For this review, take the finished solid that the model builds, in its own axes (mm). Face numbers are marked on the shaded views. A direction names the side the tool comes from. Coordinates: 2 decimals unless noted, no trailing zeros. Loops run counter-clockwise (first coordinate to the right, second up) from the corner with the lowest first, then second, coordinate; pieces in that order, holes last. Notation, with made-up numbers: M 36,-18.5 L 52,-18.5 A19 ccw 52,-12.5 Z; hole C 86.25,53.5 d8. An arc over 180 degrees is marked long. Put each result on its own line as item: value.
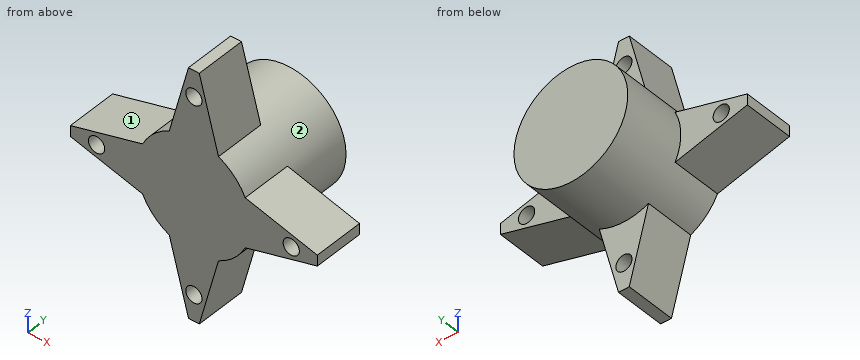
```python
from build123d import *

# Parameters (mm, degrees)
SKETCH1_R           = 7.895
BOSS_EXTRUDE1_DEPTH = 15.79
SKETCH2_R           = 1.125
BOSS_EXTRUDE2_DEPTH = 7


with BuildPart() as part:
    # Sketch1 → Boss-Extrude1 (new body)
    with BuildSketch(Plane(origin=(0, 0, 0), x_dir=(1, 0, 0), z_dir=(0, 1, 0))):
        Circle(SKETCH1_R)
    extrude(amount=BOSS_EXTRUDE1_DEPTH)

    # Sketch2 → Boss-Extrude2 (add)
    with BuildSketch(Plane(origin=(0, 0, 0), x_dir=(1, 0, 0), z_dir=(0, 1, 0))):
        Polygon((7.118925688, -3.413491182), (17.121835898, -0.746202613), (17.121835898, 0.746202613), (7.118925688, 3.413491182), (3.413491182, 7.118925688), (0.746202613, 17.121835898), (-0.746202613, 17.121835898), (-3.413491182, 7.118925688), (-7.118925688, 3.413491182), (-17.121835898, 0.746202613), (-17.121835898, -0.746202613), (-7.118925688, -3.413491182), (-3.413491182, -7.118925688), (-0.746202613, -17.121835898), (0.746202613, -17.121835898), (3.413491182, -7.118925688), align=None)
        with Locations((13.5, 0)):
            Circle(SKETCH2_R, mode=Mode.SUBTRACT)
        with Locations((0, -13.5)):
            Circle(SKETCH2_R, mode=Mode.SUBTRACT)
        with Locations((-13.5, 0)):
            Circle(SKETCH2_R, mode=Mode.SUBTRACT)
        with Locations((0, 13.5)):
            Circle(SKETCH2_R, mode=Mode.SUBTRACT)
    extrude(amount=BOSS_EXTRUDE2_DEPTH)


solid = part.part
```
(1) Add section C-C (y = 1.5). State how many separate pieces and enclosed holes the cut face has, plus the area to 3 significant figures.
Determined:
separate pieces: 1
enclosed holes: 4
area: 332 mm^2
(2) Add section D-D (z = 13.5). Write out the cut boundary in (x, y) (3 decimals), plus the area to 3 significant figures.
Determined:
outline: M -1.712,0 L -1.125,0 L -1.125,7 L -1.712,7 Z; M 1.125,0 L 1.712,0 L 1.712,7 L 1.125,7 Z
area: 8.22 mm^2
(3) Add section A-A (z = 0). Write out the cut boundary in (x, y) (3 decimals).
Determined:
outline: M -17.122,0 L -14.625,0 L -14.625,7 L -17.122,7 Z; M -12.375,0 L 12.375,0 L 12.375,7 L 7.895,7 L 7.895,15.79 L -7.895,15.79 L -7.895,7 L -12.375,7 Z; M 14.625,0 L 17.122,0 L 17.122,7 L 14.625,7 Z
(4) Wall thickness on line 1 along X through (y, z) = (2.75, 0) (3 decimals); line 2 along Z through (x, y) = (-0.5, 2.5): over which ranges is each line inside the solid? List them lowest first. Write a range as [from, to].
Determined:
line 1: x = [-17.122, -14.625], [-12.375, 12.375], [14.625, 17.122]
line 2: z = [-17.12, -14.51], [-12.49, 12.49], [14.51, 17.12]
(5) For pin 1 (2 mm diameter, centred on y = 4.5, z = -5.5, fed in from +X); pin 2 (3 mm diameter, centred on y = 10.5, z = 0.5, fed in from -X) (3 decimals); pin 3 (7.5 mm diameter, centred on x = -12.5, z = 1, fed in from +Y), all flat-tipped, find the tip position at first contact; note any pin that passes through.
Determined:
pin 1: stops at x = 6.49
pin 2: stops at x = -7.895
pin 3: stops at y = 7
(6) Tool access review of the marked faces 1 and 2: name each direction out of +Z, -Z, +X, -X, +Y, -Y from which nothing blocks a thin tool from reaching the whole face with its end or side.
Determined:
face 1: +Z, -X, +Y, -Y
face 2: +Y
(7) Add section B-B (x = -13.5). Write out the cut boundary in (y, z) (3 decimals).
Determined:
outline: M 0,-1.712 L 7,-1.712 L 7,-1.125 L 0,-1.125 Z; M 0,1.125 L 7,1.125 L 7,1.712 L 0,1.712 Z
